Part model, mm, in its own coordinate system. A direction names the side the tool comes from. Give positions to 0.01 mm unless a question says otherwise; leave off trailing zeros. Write each loop counter-clockwise with the first axis right and the second up, starting at its lowest first coordinate (ties: lowest second). Pieces come first, ordered by that corner, then holes. Notation, with made-up numbers: (78.5, 26) - (94.5, 26) arc R9 cw to (94.5, 38) - close; hole circle Ø1 at (-18.5, 35). An arc over 180 degrees is marked (long way). Answer as a JSON object with one key per item and string values. Group by question number.
```python
from build123d import *

# Parameters (mm, degrees)
EXTRUDE_1_DEPTH          = 18
CUT_EXTRUDE_1_DEPTH      = 19
HOLE_WIZARD_M3_1_D       = 3.6
PATTERN_CIRCULAR_1_COUNT = 8


with BuildPart() as part:
    # ｽｹｯﾁ1 → ﾎﾞｽ - 押し出し1 (new body)
    with BuildSketch(Plane.XY):
        with BuildLine():
            ThreePointArc((-31, 0), (0, 31), (31, 0))
            Line((31, 0), (31, -11))
            Line((31, -11), (-31, -11))
            Line((-31, -11), (-31, 0))
        make_face()
    extrude(amount=EXTRUDE_1_DEPTH)

    # ｽｹｯﾁ2 → ｶｯﾄ - 押し出し1 (cut, through all)
    with BuildSketch(Plane.XY.offset(18)):
        with BuildLine():
            Line((-24, 0), (-24, -11))
            Line((-24, -11), (24, -11))
            Line((24, -11), (24, 0))
            ThreePointArc((24, 0), (0, 24), (-24, 0))
        make_face()
    extrude(amount=-CUT_EXTRUDE_1_DEPTH, mode=Mode.SUBTRACT)

    # M3 すきま穴1 (through all)
    with Locations(Plane.XY.offset(18)):
        with Locations((0, 27.5)):
            hole_wizard_m3_1 = Hole(HOLE_WIZARD_M3_1_D / 2)

    # 円形ﾊﾟﾀｰﾝ1: M3 すきま穴1 ×8 about axis, 3 skipped
    pattern_circular_1_axis = Axis((0, 0, 0), (0, 0, -1))
    add([hole_wizard_m3_1.rotate(pattern_circular_1_axis, i * 360 / PATTERN_CIRCULAR_1_COUNT) for i in range(1, PATTERN_CIRCULAR_1_COUNT) if i not in (3, 4, 5)], mode=Mode.SUBTRACT)


solid = part.part
```
1) Drop flat-ended pins along their axis: P1, Ø5, axis at y = 6, z = 2.5, coming from the +X side; P2, Ø8, axis at x = 7.5, z = 8, coming from the -Y side; P3, Ø3, axis at x = 27.5, y = 0, coming from the +Z side; P4, Ø2, axis at x = 11.5, z = 7, coming from the -Y side. Give the stop position or say it passes through.
2) Saw through at A-A (x = 0). List the corners of the cut face in (y, z).
3) Saw through at D-D (x = -10.5). List the corners of the cut face in (y, z), and give its area (3 significant figures).
4) Which spindle directions (+Z, -Z, +X, -X, +Y, -Y) get a long thin tool onto all of the face, cutting with end or side? Do faces 4 (the flat face through (-31, -6, 9)), 5 (the flat face through (24, -6, 9)). Say none if no direction does.
5) Two-plate mould, pull along Y, no slides. Class faces 1 (the flat face through (28, -11, 9)), 2 (the cylindrical face through (0.234, 29.285, 8.874)), 3 (the flat face through (-24, -5, 9)): +Y half, -Y half, draft (parallel to the pull), parting line (faces both ways), or undercut.
6) Saw through at C-C (z = 13.75). List the corners of the cut face in (x, y), and give its area (3 significant figures).
7) Drill centre lines: line 1 along X through (y, z) = (18, 11.75); line 2 along X through (y, z) = (-1.5, 9); line 3 along Y through (x, z) = (-0.5, 17). Where is each one in solid material? Low to high. Write a range as from..to.
8) Saw through at B-B (y = -4). List the corners of the cut face in (x, z), and give its area (3 significant figures).
Checks:
{
 "1": {"P1": "x = 30.8", "P2": "y = 21.07", "P3": "through", "P4": "y = 20.49"},
 "2": {"outline": "(24, 0) - (25.7, 0) - (25.7, 18) - (24, 18) - close; (29.3, 0) - (31, 0) - (31, 18) - (29.3, 18) - close"},
 "3": {"outline": "(21.58, 0) - (29.17, 0) - (29.17, 18) - (21.58, 18) - close", "area": "137 mm2"},
 "4": {"face 4": "+Z, -Z, -X, +Y, -Y", "face 5": "+Z, -Z, -Y"},
 "5": {"face 1": "-Y half", "face 2": "undercut", "face 3": "draft"},
 "6": {"outline": "(-31, -11) - (-24, -11) - (-24, 0) arc R24 cw to (24, 0) - (24, -11) - (31, -11) - (31, 0) arc R31 ccw to (-31, 0) - close; hole circle Ø3.6 at (-27.5, 0); hole circle Ø3.6 at (-19.45, 19.45); hole circle Ø3.6 at (0, 27.5); hole circle Ø3.6 at (19.45, 19.45); hole circle Ø3.6 at (27.5, 0)", "area": "708 mm2"},
 "7": {"line 1": "-25.24..-20.52, -18.37..-15.87, 15.87..18.37, 20.52..25.24", "line 2": "-31..-28.49, -26.51..-24, 24..26.51, 28.49..31", "line 3": "23.99..25.77, 29.23..31"},
 "8": {"outline": "(-31, 0) - (-24, 0) - (-24, 18) - (-31, 18) - close; (24, 0) - (31, 0) - (31, 18) - (24, 18) - close", "area": "252 mm2"}
}
